from build123d import *

# Parameters (mm, degrees)
BOSS_EXTRUDE2_DEPTH = 0.3175
SKETCH3_R           = 4.2
SKETCH3_W           = 25.956624075
SKETCH3_H           = 5
CUT_EXTRUDE1_DEPTH  = 1.3175


with BuildPart() as part:
    # Sketch2 → Boss-Extrude2 (new body)
    with BuildSketch(Plane.XY):
        with BuildLine():
            Line((-6.375715531, -5.168393782), (-6.375715531, 4.831606218))
            Line((-6.375715531, 4.831606218), (-7.593127245, 4.831606218))
            ThreePointArc((-7.593127245, 4.831606218), (-8.997720551, -0.202546003), (-7.368019117, -5.168393782))
            Line((-7.368019117, -5.168393782), (-6.375715531, -5.168393782))
        make_face()
        with BuildLine():
            Line((-7.593127245, 4.831606218), (-6.375715531, 4.831606218))
            Line((-6.375715531, 4.831606218), (-6.375715531, -5.168393782))
            Line((-6.375715531, -5.168393782), (-7.368019117, -5.168393782))
            ThreePointArc((-7.368019117, -5.168393782), (2.709965677, -8.582312394), (9, 0))
            ThreePointArc((9, 0), (2.516133422, 8.641126813), (-7.593127245, 4.831606218))
        make_face()
        with BuildLine():
            ThreePointArc((-7.368019117, -5.168393782), (-8.997720551, -0.202546003), (-7.593127245, 4.831606218))
            Line((-7.593127245, 4.831606218), (-41.375715531, 4.831606218))
            Line((-41.375715531, 4.831606218), (-41.375715531, -5.168393782))
            Line((-41.375715531, -5.168393782), (-7.368019117, -5.168393782))
        make_face()
    extrude(amount=BOSS_EXTRUDE2_DEPTH)

    # Sketch3 → Cut-Extrude1 (cut, through all)
    with BuildSketch(Plane.XY.offset(0.3175)):
        Circle(SKETCH3_R)
        with Locations((-20.034010662, 0.207958654)):
            Rectangle(SKETCH3_W, SKETCH3_H)
    extrude(amount=-CUT_EXTRUDE1_DEPTH, mode=Mode.SUBTRACT)


solid = part.part
Check sheet for the modelled part. Datum: model origin and axes. Units: mm. Round coordinates to 2 decimals unless told otherwise and drop trailing zeros. Loops run counter-clockwise (first coordinate to the right, second up) from the corner with the lowest first, then second, coordinate; pieces in that order, holes last. Notation, with made-up numbers: (45, -6.5) -> (63, -6.5) arc R22 cw to (63, 11.5) -> close; hole circle Ø4 at (-36, 54). An arc over 180 degrees is marked (long way). Put each result on its own line as item: value. Start each with the question number.
1. Section check D-D (x = -5.5). Enter the section's corners in (y, z), plus the area to 3 significant figures.
2. Section check C-C (y = -2.75). Enter the section's corners in (x, z), plus the area to 3 significant figures.
3. Scan lines: probe 1 along X at (y, z) = (-1, 0.25); probe 2 along Y at (x, z) = (0, 0.1); probe 3 along Y at (x, z) = (-13.5, 0.1). Record each from-to range of solid material in increasing order.
4. Draft check along X on faces 1 (the face through (4.006, 1.262, 0.161)), 2 (the face through (-17, 4, 0)). Enter one of: +X half, -X half, draft (parallel to the pull), parting line (faces both ways), or undercut.
5. Section check B-B (z = 0.25). Enter the section's corners in (x, y).
6. Gauge pin test, flat end, axial feed: pin 1 (1 mm diameter, centred on x = -21, y = -0.5, fed in from -Z). Record the tip position at first contact, or that the pin passes through.
7. Section check A-A (x = -18.5). Enter the section's corners in (y, z).
Findings:
1. outline: (-7.12, 0) -> (7.12, 0) -> (7.12, 0.32) -> (-7.12, 0.32) -> close
1. area: 4.52 mm^2
2. outline: (-41.38, 0) -> (-3.17, 0) -> (-3.17, 0.32) -> (-41.38, 0.32) -> close; (3.17, 0) -> (8.57, 0) -> (8.57, 0.32) -> (3.17, 0.32) -> close
2. area: 13.8 mm^2
3. probe 1: x = -41.38 to -33.01, -7.06 to -4.08, 4.08 to 8.94
3. probe 2: y = -9 to -4.2, 4.2 to 9
3. probe 3: y = -5.17 to -2.29, 2.71 to 4.83
4. face 1: undercut
4. face 2: draft
5. outline: (-41.38, -5.17) -> (-7.37, -5.17) arc R9 ccw (long way) to (-7.59, 4.83) -> (-41.38, 4.83) -> close; hole (-33.01, -2.29) -> (-7.06, -2.29) -> (-7.06, 2.71) -> (-33.01, 2.71) -> close; hole circle Ø8.4 at (0, 0)
6. pin 1: passes through
7. outline: (-5.17, 0) -> (-2.29, 0) -> (-2.29, 0.32) -> (-5.17, 0.32) -> close; (2.71, 0) -> (4.83, 0) -> (4.83, 0.32) -> (2.71, 0.32) -> close
